Verification items for the finished model (mm, model axes). A direction names the side the tool comes from. Round coordinates to 2 decimals unless told otherwise and drop trailing zeros. Loops run counter-clockwise (first coordinate to the right, second up) from the corner with the lowest first, then second, coordinate; pieces in that order, holes last. Notation, with made-up numbers: (-14, 2) - (44, 2) arc R22 cw to (44, 39) - close; hole circle Ø6 at (46, 40). An arc over 180 degrees is marked (long way). Use a Markdown table: item, result. Add a question column.
```python
from build123d import *

# Parameters (mm, degrees)
SKETCH_W     = 20
SKETCH_H     = 20
PAD_DEPTH    = 20
SKETCH001_W  = 15
SKETCH001_H  = 15
POCKET_DEPTH = 17.5
FILLET_R     = 1


with BuildPart() as part:
    # Sketch → Pad (new body)
    with BuildSketch(Plane.XY):
        Rectangle(SKETCH_W, SKETCH_H)
    extrude(amount=PAD_DEPTH)

    # Sketch001 (on Face6 of Pad) → Pocket (cut)
    with BuildSketch(Plane.XY.offset(20)):
        Rectangle(SKETCH001_W, SKETCH001_H)
    extrude(amount=-POCKET_DEPTH, mode=Mode.SUBTRACT)

    # Fillet
    fillet_edges = [part.edges().sort_by_distance(p)[0] for p in [
        (-10, 0, 0),
        (-10, -10, 10),
        (-10, 10, 10),
        (0, 10, 0),
        (10, 0, 0),
        (0, -10, 0),
        (10, -10, 10),
        (10, 10, 10),
        (10, 0, 20),
        (0, 10, 20),
        (0, 7.5, 20),
        (7.5, 0, 2.5),
        (7.5, 0, 20),
        (0, -7.5, 20),
        (0, -10, 20),
        (-10, 0, 20),
        (0, -7.5, 2.5),
        (-7.5, 0, 20),
        (7.5, -7.5, 11.25),
        (7.5, 7.5, 11.25),
        (0, 7.5, 2.5),
        (-7.5, 7.5, 11.25),
        (-7.5, 0, 2.5),
        (-7.5, -7.5, 11.25),
    ]]
    fillet(fillet_edges, radius=FILLET_R)


solid = part.part
```
Q1. Section check D-D on z = 3. Record the cut outline in (x, y).
Q2. Set-up check for faces 4 (the face through (-9.715, -9.699, 10.126)), 5 (the face through (-7.5, 0, 11)): record each of +Z, -Z, +X, -X, +Y, -Y from which the full face is reachable in a straight line by a thin tool's end or side.
Q3. Thickness scan on line 1 along X through (y, z) = (-5, 18.25); line 2 along Z through (x, y) = (-4, -5.25). Record the ranges inside material, lowest first.
Q4. Go/stop test with flat-tipped pins: pin 1 Ø2 at (x, y) = (4, -3) entering from +Z; pin 2 Ø10.5 at (x, y) = (2, 0) entering from +Z. Record where each tip stops, or that it passes through.
Q5. Section check B-B on x = -5. Record the cut outline in (y, z), plus the area to 3 significant figures.
Q6. Section check A-A on z = 13. Record the cut outline in (x, y).
Q7. Release check for a two-part mould opening along Y. For faces 1 (the face through (0, -10, 10)), 2 (the face through (0, 7.5, 11)), 3 (the face through (-9.715, 9.699, 10.126)) record: +Y half, -Y half, draft (parallel to the pull), parting line (faces both ways), or undercut.
Determined:
| question | item | result |
|---|---|---|
| 1 | outline | (-10, -9) arc R1 ccw to (-9, -10) - (9, -10) arc R1 ccw to (10, -9) - (10, 9) arc R1 ccw to (9, 10) - (-9, 10) arc R1 ccw to (-10, 9) - close; hole (-7.37, -6.5) arc R0.87 ccw to (-6.5, -7.37) - (6.5, -7.37) arc R0.87 ccw to (7.37, -6.5) - (7.37, 6.5) arc R0.87 ccw to (6.5, 7.37) - (-6.5, 7.37) arc R0.87 ccw to (-7.37, 6.5) - close |
| 2 | face 4 | +Z, -Z, -X, -Y |
| 2 | face 5 | +Z |
| 3 | line 1 | x = -10 to -7.5, 7.5 to 10 |
| 3 | line 2 | z = 0 to 2.5 |
| 4 | pin 1 | stops at z = 2.5 |
| 4 | pin 2 | stops at z = 2.84 |
| 5 | outline | (-10, 1) arc R1 ccw to (-9, 0) - (9, 0) arc R1 ccw to (10, 1) - (10, 19) arc R1 ccw to (9, 20) - (8.5, 20) arc R1 ccw to (7.5, 19) - (7.5, 3.5) arc R1 cw to (6.5, 2.5) - (-6.5, 2.5) arc R1 cw to (-7.5, 3.5) - (-7.5, 19) arc R1 ccw to (-8.5, 20) - (-9, 20) arc R1 ccw to (-10, 19) - close |
| 5 | area | 137 mm² |
| 6 | outline | (-10, -9) arc R1 ccw to (-9, -10) - (9, -10) arc R1 ccw to (10, -9) - (10, 9) arc R1 ccw to (9, 10) - (-9, 10) arc R1 ccw to (-10, 9) - close; hole (-7.5, -6.5) arc R1 ccw to (-6.5, -7.5) - (6.5, -7.5) arc R1 ccw to (7.5, -6.5) - (7.5, 6.5) arc R1 ccw to (6.5, 7.5) - (-6.5, 7.5) arc R1 ccw to (-7.5, 6.5) - close |
| 7 | face 1 | -Y half |
| 7 | face 2 | undercut |
| 7 | face 3 | +Y half |
